Work out the finished part from the listing and answer in its coordinate system (mm). Coordinates: 2 decimals unless noted, no trailing zeros. Answer in a Markdown table with one row per item. Add a question column.
Item 1: Flat-ended cylindrical pins translate along their axes: pin 1 Ø0.6 at (x, z) = (-172.5, 1.5) entering from -Y; pin 2 Ø0.6 at (y, z) = (-168, 1.5) entering from -X; pin 3 Ø1 at (y, z) = (-198, 1) entering from -X. Find the tip coordinate at first contact, or state that the pin passes through.
Item 2: Consider line 1 (X direction, y = -161.5, z = 2.9); line 2 (X direction, y = -191, z = 2.85); line 3 (Y direction, x = -131.5, z = 0.5). Determine where each line is inside the solid, lowest interval first. Write a range as from..to.
Item 3: The mould has two halves that part along Z. Classify faces 1 (the face through (45, -180, 0)), 2 (the face through (45, -180, 3.175)): released by +Z, released by -Z, zero draft, split by the parting line, or undercut.
from build123d import *

# Parameters (mm, degrees)
BOSS_EXTRUDE1_DEPTH = 3.175


with BuildPart() as part:
    # Sketch2 → Boss-Extrude1 (new body)
    with BuildSketch(Plane.XY):
        with BuildLine():
            Line((249.446820082, -203.714000022), (249.446820082, -194.181000022))
            Line((249.446820082, -194.181000022), (267.623820082, -194.181000022))
            Line((267.623820082, -194.181000022), (267.623820082, -193.665000022))
            Line((267.623820082, -193.665000022), (268.766820082, -193.665000022))
            Line((268.766820082, -193.665000022), (268.766820082, -168.265000022))
            Line((268.766820082, -168.265000022), (267.623820082, -168.265000022))
            Line((267.623820082, -168.265000022), (267.623820082, -167.122000022))
            Line((267.623820082, -167.122000022), (269.766820082, -167.122000022))
            Line((269.766820082, -167.122000022), (269.766820082, -157.216000022))
            Line((269.766820082, -157.216000022), (240.172195086, -157.216000021))
            Line((240.172195086, -157.216000021), (240.172195086, -161.66050002))
            ThreePointArc((240.172195086, -161.66050002), (239.707227101, -162.783032036), (238.584695086, -163.24800002))
            Line((238.584695086, -163.24800002), (230.695695086, -163.24800002))
            ThreePointArc((230.695695086, -163.24800002), (229.573163071, -162.783032035), (229.108195086, -161.66050002))
            Line((229.108195086, -161.66050002), (229.108195086, -157.216000021))
            Line((229.108195086, -157.216000021), (138.573445094, -157.216000021))
            Line((138.573445094, -157.216000021), (138.573445094, -161.66050002))
            ThreePointArc((138.573445094, -161.66050002), (138.108477109, -162.783032035), (136.985945094, -163.24800002))
            Line((136.985945094, -163.24800002), (129.096945094, -163.24800002))
            ThreePointArc((129.096945094, -163.24800002), (127.974413079, -162.783032035), (127.509445094, -161.66050002))
            Line((127.509445094, -161.66050002), (127.509445094, -157.216000021))
            Line((127.509445094, -157.216000021), (58.558195094, -157.216000021))
            Line((58.558195094, -157.216000021), (58.558195094, -161.66050002))
            ThreePointArc((58.558195094, -161.66050002), (58.093227109, -162.783032035), (56.970695094, -163.24800002))
            Line((56.970695094, -163.24800002), (49.081695094, -163.24800002))
            ThreePointArc((49.081695094, -163.24800002), (47.959163079, -162.783032035), (47.494195094, -161.66050002))
            Line((47.494195094, -161.66050002), (47.494195094, -157.216000021))
            Line((47.494195094, -157.216000021), (-43.040554898, -157.21600002))
            Line((-43.040554898, -157.21600002), (-43.040554898, -161.660500019))
            ThreePointArc((-43.040554898, -161.660500019), (-43.505522883, -162.783032034), (-44.628054898, -163.248000019))
            Line((-44.628054898, -163.248000019), (-52.517054898, -163.248000019))
            ThreePointArc((-52.517054898, -163.248000019), (-53.639586913, -162.783032034), (-54.104554898, -161.660500019))
            Line((-54.104554898, -161.660500019), (-54.104554898, -157.21600002))
            Line((-54.104554898, -157.21600002), (-123.055804898, -157.21600002))
            Line((-123.055804898, -157.21600002), (-123.055804898, -161.660500019))
            ThreePointArc((-123.055804898, -161.660500019), (-123.520772883, -162.783032034), (-124.643304898, -163.248000019))
            Line((-124.643304898, -163.248000019), (-132.532304898, -163.248000019))
            ThreePointArc((-132.532304898, -163.248000019), (-133.654836913, -162.783032034), (-134.119804898, -161.660500019))
            Line((-134.119804898, -161.660500019), (-134.119804898, -157.21600002))
            Line((-134.119804898, -157.21600002), (-174.499179878, -157.21600002))
            Line((-174.499179878, -157.21600002), (-174.499179878, -167.12200002))
            Line((-174.499179878, -167.12200002), (-172.356179878, -167.12200002))
            Line((-172.356179878, -167.12200002), (-172.356179878, -168.26500002))
            Line((-172.356179878, -168.26500002), (-173.499179878, -168.26500002))
            Line((-173.499179878, -168.26500002), (-173.499179878, -193.66500002))
            Line((-173.499179878, -193.66500002), (-172.356179878, -193.66500002))
            Line((-172.356179878, -193.66500002), (-172.356179878, -194.18100002))
            Line((-172.356179878, -194.18100002), (-154.179179878, -194.18100002))
            Line((-154.179179878, -194.18100002), (-154.179179878, -203.71400002))
            Line((-154.179179878, -203.71400002), (249.446820082, -203.714000022))
        make_face()
    extrude(amount=BOSS_EXTRUDE1_DEPTH)


solid = part.part
Reply:
| question | item | result |
|---|---|---|
| 1 | pin 1 | stops at y = -194.18 |
| 1 | pin 2 | stops at x = -173.5 |
| 1 | pin 3 | stops at x = -154.18 |
| 2 | line 1 | x = -174.5..-134.12, -123.06..-54.1, -43.04..47.49, 58.56..127.51, 138.57..229.11, 240.17..269.77 |
| 2 | line 2 | x = -173.5..268.77 |
| 2 | line 3 | y = -203.71..-163.25 |
| 3 | face 1 | released by -Z |
| 3 | face 2 | released by +Z |
